Design review of the part built by this model. Coordinates are the model's own, in mm. Face numbers are marked on the shaded views. A direction names the side the tool comes from. Coordinates: 2 decimals unless noted, no trailing zeros. Write each loop counter-clockwise with the first axis right and the second up, starting at its lowest first coordinate (ties: lowest second). Pieces come first, ordered by that corner, then holes.
Autodesk Fusion 360 part; units mm, degrees
sketch "Schizzo1" plane through (0, 0, 0) normal (0, 0, 1) x (1, 0, 0)
  line L0 (0, 0) -> (13, 0)
  line L1 (13, 0) -> (13, 8)
  line L2 (13, 8) -> (0, 8)
  line L3 (0, 8) -> (0, 0)
  line L4 (0, -5) -> (-4.3713, -5)
  line L5 (-4.3713, -5) -> (-4.3713, 13)
  line L6 (-4.3713, 13) -> (0, 13)
  line L7 (0, 13) -> (0, -5)
  dimension "d1" = 13
  dimension "d2" = 8
  dimension "d3" = 5
  dimension "d4" = 5
extrude "Estrusione1" add sketch "Schizzo1" along normal blind 6.5 makes body 1
chamfer "Smusso1" distance 3.5 angle 45 2 edges at (-4.3713, -5, 3.25) (-4.3713, 13, 3.25) on bodies 1
extrude "Estrusione2" add sketch "Schizzo1" along normal blind 8 separate body makes body 2
chamfer "Smusso2" distance 2 angle 45 2 edges at (-4.3713, -5, 4) (-4.3713, 13, 4) on bodies 2
chamfer "Smusso3" distance 2.5 angle 45 1 edges at (13, 4, 8) on bodies 2
hidden bodies 1
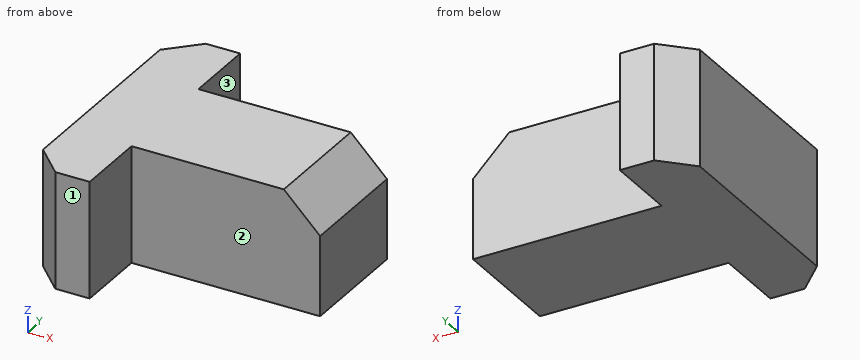
(1) Consider section D-D (z = 4.5). Give the boundary of the cut face in (x, y).
(2) For the marked faces 1, 2 and 3, list the 3-axis set-ups (+Z, -Z, +X, -X, +Y, -Y) from which the entire face can be reached by the end or side of a thin tool; tool diameter is ignored.
(3) Insertion check: pin 1 Ø2.5 at (y, z) = (-3.5, 2.5) entering from +X; pin 2 Ø2.5 at (x, z) = (9.5, 3) entering from +Y. Each pin has a flat end and moves straight along its axis. Give the tip position at first contact, or say it passes through.
(4) Wall thickness on line 1 (Y direction, x = 7.5, z = 1.25); line 2 (X direction, y = 9.5, z = 5); line 3 (Y direction, x = -3.25, z = 4.75): over which ranges is each line inside the solid? List them lowest first.
(5) Consider section B-B (x = 3). Give the boundary of the cut face in (y, z).
(6) Consider section C-C (y = 2.25). Give the boundary of the cut face in (x, z).
(7) Consider section A-A (z = 5.75). Give the boundary of the cut face in (x, y), plus the area to 3 significant figures.
Results:
1. outline: (-4.37, -3) - (-2.37, -5) - (0, -5) - (0, 0) - (13, 0) - (13, 8) - (0, 8) - (0, 13) - (-2.37, 13) - (-4.37, 11) - close
2. face 1: +Z, -Z, +X, -X, -Y
2. face 2: +Z, -Z, +X, -Y
2. face 3: +Z, -Z, +X, +Y
3. pin 1: stops at x = 0
3. pin 2: stops at y = 8
4. line 1: y = 0 to 8
4. line 2: x = -4.37 to 0
4. line 3: y = -4.12 to 12.12
5. outline: (0, 0) - (8, 0) - (8, 8) - (0, 8) - close
6. outline: (-4.37, 0) - (13, 0) - (13, 5.5) - (10.5, 8) - (-4.37, 8) - close
7. outline: (-4.37, -3) - (-2.37, -5) - (0, -5) - (0, 0) - (12.75, 0) - (12.75, 8) - (0, 8) - (0, 13) - (-2.37, 13) - (-4.37, 11) - close
7. area: 177 mm2
